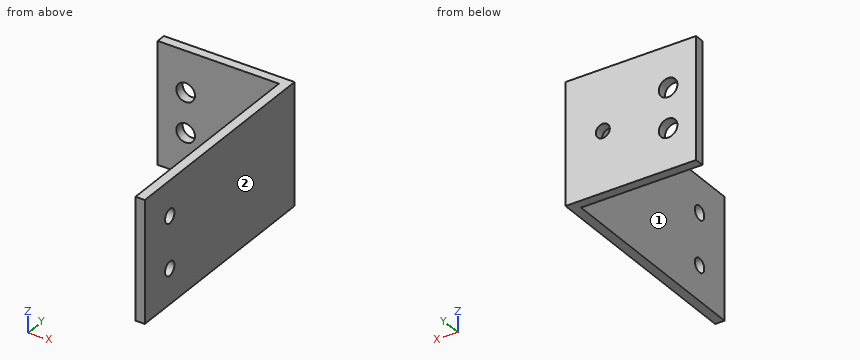
from build123d import *

# Parameters (mm, degrees)
F1_DEPTH = 41.275
F2_R     = 4.7625
F3_DEPTH = 88.901
F4_R     = 6.35
F4_R_2   = 4.7625
F5_DEPTH = 152.401


with BuildPart() as f1:
    # F0 (on Top) → F1 (new body, symmetric)
    with BuildSketch(Plane.XY):
        Polygon((-82.55, 0), (0, 0), (0, -146.05), (6.35, -146.05), (6.35, 6.35), (-82.55, 6.35), align=None)
    extrude(amount=F1_DEPTH, both=True)

    # F2 (on face) → F3 (cut, through all)
    with BuildSketch(Plane.YZ.offset(6.35)):
        with Locations((-120.65, 17.4625)):
            Circle(F2_R)
        with Locations((-120.65, -17.4625)):
            Circle(F2_R)
    extrude(amount=-F3_DEPTH, mode=Mode.SUBTRACT)

    # F4 (on face) → F5 (cut, through all)
    with BuildSketch(Plane(origin=(0, 6.35, 0), x_dir=(-1, 0, 0), z_dir=(0, 1, 0))):
        with Locations((63.5, 13.4874)):
            Circle(F4_R)
        with Locations((63.5, -13.4874)):
            Circle(F4_R)
        with Locations((19.05, 0)):
            Circle(F4_R_2)
    extrude(amount=-F5_DEPTH, mode=Mode.SUBTRACT)


solid = f1.part
Design review of the part built by this model. Coordinates are the model's own, in mm. Face numbers are marked on the shaded views. A direction names the side the tool comes from. Round coordinates to 2 decimals unless told otherwise and drop trailing zeros. Write each loop counter-clockwise with the first axis right and the second up, starting at its lowest first coordinate (ties: lowest second). Pieces come first, ordered by that corner, then holes. Notation, with made-up numbers: M 31,-10.75 L 41,-10.75 A23 cw 41,13.25 Z; hole C -34,-35 d10. An arc over 180 degrees is marked long. One line per item, written item: value. Start each with the question number.
1. To check wall thickness, follow probe 1 along Z at (x, y) = (3.75, -120.65) (3 decimals); probe 2 along Z at (x, y) = (-63, 3) (3 decimals); probe 3 along Z at (x, y) = (-19.05, 2.75) (1 decimal). State the ranges of each line that lie inside material, in increasing order. Write a range as from..to.
2. For the marked faces 1 and 2, list the 3-axis set-ups (+Z, -Z, +X, -X, +Y, -Y) from which the entire face can be reached by the end or side of a thin tool; tool diameter is ignored.
3. Take a section at C-C on z = 0. State the section outline as (x, y) points, then the cut area to 3 significant figures.
4. Take a section at A-A on y = -120.65. State the section outline as (x, z) points (3 decimals), then the cut area to 3 significant figures.
5. Take a section at D-D on x = -63.5. State the section outline as (y, z) points (3 decimals), then the cut area to 3 significant figures.
6. Clearance check with flat-ended pins moving along their axes: P1, Ø16.5, axis at x = -63.5, z = -13.49, coming from the -Y side; P2, Ø5.5, axis at y = -120.65, z = -17.46, coming from the -X side. State where each tip first meets the part, or that it passes through.
Computed:
1. probe 1: z = -41.275..-22.225, -12.7..12.7, 22.225..41.275
1. probe 2: z = -41.275..-19.818, -7.157..7.157, 19.818..41.275
1. probe 3: z = -41.3..-4.8, 4.8..41.3
2. face 1: +Z, -Z, -X, -Y
2. face 2: +Z, -Z, +X, +Y, -Y
3. outline: M -82.55,0 L -23.81,0 L -23.81,6.35 L -82.55,6.35 Z; M -14.29,0 L 0,0 L 0,-146.05 L 6.35,-146.05 L 6.35,6.35 L -14.29,6.35 Z
3. area: 1,430 mm²
4. outline: M 0,-41.275 L 6.35,-41.275 L 6.35,-22.225 L 0,-22.225 Z; M 0,-12.7 L 6.35,-12.7 L 6.35,12.7 L 0,12.7 Z; M 0,22.225 L 6.35,22.225 L 6.35,41.275 L 0,41.275 Z
4. area: 403 mm²
5. outline: M 0,-41.275 L 6.35,-41.275 L 6.35,-19.837 L 0,-19.837 Z; M 0,-7.137 L 6.35,-7.137 L 6.35,7.137 L 0,7.137 Z; M 0,19.837 L 6.35,19.837 L 6.35,41.275 L 0,41.275 Z
5. area: 363 mm²
6. P1: stops at y = 0
6. P2: passes through
